from build123d import *

# Parameters (mm, degrees)
F1_DEPTH = 145
F2_T     = -2.5
F4_DEPTH = 145
F6_D     = 8


# Not quite as in the source:
# - a feature names something its author has since deleted; it is built from what else it names


with BuildPart() as f1:
    # F0 (on Right) → F1 (new body)
    with BuildSketch(Plane.YZ):
        Polygon((109.173472161, 35), (-70.826527839, 55), (-70.826527839, 0), (109.173472161, 0), align=None)
    extrude(amount=F1_DEPTH)

    # F2
    f2_openings = [f1.faces().sort_by_distance(p)[0] for p in [
        (72.5, -70.826528, 27.5),
    ]]
    offset(amount=F2_T, openings=f2_openings)

    # F3 (on face) → F4 (cut)
    with BuildSketch(Plane.YZ.offset(145)):
        Polygon((94.173472161, 36.6666666667), (-35.826527839, 51.1111111111), (-35.826527839, 20), (94.173472161, 20), align=None)
    extrude(amount=-F4_DEPTH, mode=Mode.SUBTRACT)

    # F6 (through all)
    with Locations(Plane(origin=(0, 0, 0), x_dir=(1, 0, 0), z_dir=(0, 0, -1))):
        with Locations((109.5, 20.826527839), (35.5, 20.826527839), (35.5, -53.173472161), (109.5, -53.173472161)):
            Hole(F6_D / 2)


solid = f1.part
Input: part model. Units: mm. Frame: model coordinates. A direction names the side the tool comes from. Coordinates: 2 decimals unless noted, no trailing zeros. Loops run counter-clockwise (first coordinate to the right, second up) from the corner with the lowest first, then second, coordinate; pieces in that order, holes last. Notation, with made-up numbers: (65.5, -1.5) -> (99.5, -1.5) arc R15 ccw to (99.5, 27.5) -> close; hole circle Ø11 at (18.25, 41). An arc over 180 degrees is marked (long way). Write item = value, one per line. Start each with the question number.
Item 1: Cut plane B-B, the plane z = 23. Return loops of the section in (x, y), plus the area to 3 significant figures.
Item 2: Mould query, pull axis Z, two halves, no side actions, for faces 1 (the face through (142.5, -3, 17)), 2 (the face through (71.52, -53.082, 50.513)), 3 (the face through (71.48, 101.78, 35.82)), 4 (the face through (51, -70.827, 1)). Classes: pulls with the +Z half, pulls with the -Z half, needs draft (parallel to the pull), parting line crosses it, or undercut.
Item 3: Cut plane D-D, the plane z = 44.5. Return loops of the section in (x, y), plus the area to 3 significant figures.
Item 4: First-contact query: P1, Ø13, axis at x = 35.5, y = -20.83, coming from the +Z side; P2, Ø2, axis at x = 42, z = 24, coming from the -Y side; P3, Ø3, axis at x = 143.5, y = 54.5, coming from the +Z side; P4, Ø6, axis at x = 56.5, z = 41, coming from the -Y side. Flat tips, straight axial feed; report the tip coordinate or a pass-through.
Item 5: Cut plane A-A, the plane x = 35.5. Return loops of the section in (y, z), plus the area to 3 significant figures.
Item 6: Reachability of faces 5 (the face through (110.367, -16.922, 1.268)), 6 (the face through (72, 17, 2.5)), 7 (the face through (84, 94.173, 35)) from +Z, -Z, +X, -X, +Y, -Y: full face, straight path, thin tool, end or side. Return the list, or none.
Item 7: Cut plane C-C, the plane x = 64. Return loops of the section in (y, z), plus the area to 3 significant figures.
Item 8: Material intervals for line 1 (Y direction, x = 35.5, z = 1.55); line 2 (Y direction, x = 109, z = 1); line 3 (X direction, y = 95.5, z = 25), sorted ascending.
Ans:
q1.outline = (0, -70.83) -> (2.5, -70.83) -> (2.5, -35.83) -> (0, -35.83) -> close; (0, 94.17) -> (2.5, 94.17) -> (2.5, 106.67) -> (142.5, 106.67) -> (142.5, 94.17) -> (145, 94.17) -> (145, 109.17) -> (0, 109.17) -> close; (142.5, -70.83) -> (145, -70.83) -> (145, -35.83) -> (142.5, -35.83) -> close
q1.area = 600 mm²
q2.face_1 = undercut
q2.face_2 = undercut
q2.face_3 = pulls with the +Z half
q2.face_4 = needs draft
q3.outline = (0, -70.83) -> (2.5, -70.83) -> (2.5, -35.83) -> (0, -35.83) -> close; (142.5, -70.83) -> (145, -70.83) -> (145, -35.83) -> (142.5, -35.83) -> close
q3.area = 175 mm²
q4.P1 = 2.5
q4.P2 = 106.67
q4.P3 = 20
q4.P4 = through
q5.outline = (-70.83, 0) -> (-24.83, 0) -> (-24.83, 2.5) -> (-70.83, 2.5) -> close; (-70.83, 52.48) -> (-35.83, 48.6) -> (-35.83, 51.11) -> (-70.83, 55) -> close; (-16.83, 0) -> (49.17, 0) -> (49.17, 2.5) -> (-16.83, 2.5) -> close; (57.17, 0) -> (109.17, 0) -> (109.17, 35) -> (94.17, 36.67) -> (94.17, 34.15) -> (106.67, 32.76) -> (106.67, 2.5) -> (57.17, 2.5) -> close
q5.area = 611 mm²
q6.face_5 = +Z, -Z
q6.face_6 = -Y
q6.face_7 = +Z, +X, -X
q7.outline = (-70.83, 0) -> (109.17, 0) -> (109.17, 35) -> (94.17, 36.67) -> (94.17, 34.15) -> (106.67, 32.76) -> (106.67, 2.5) -> (-70.83, 2.5) -> close; (-70.83, 52.48) -> (-35.83, 48.6) -> (-35.83, 51.11) -> (-70.83, 55) -> close
q7.area = 651 mm²
q8.line_1 = -70.83 to -24.83, -16.83 to 49.17, 57.17 to 109.17
q8.line_2 = -70.83 to -24.8, -16.86 to 49.2, 57.14 to 109.17
q8.line_3 = 0 to 2.5, 142.5 to 145
